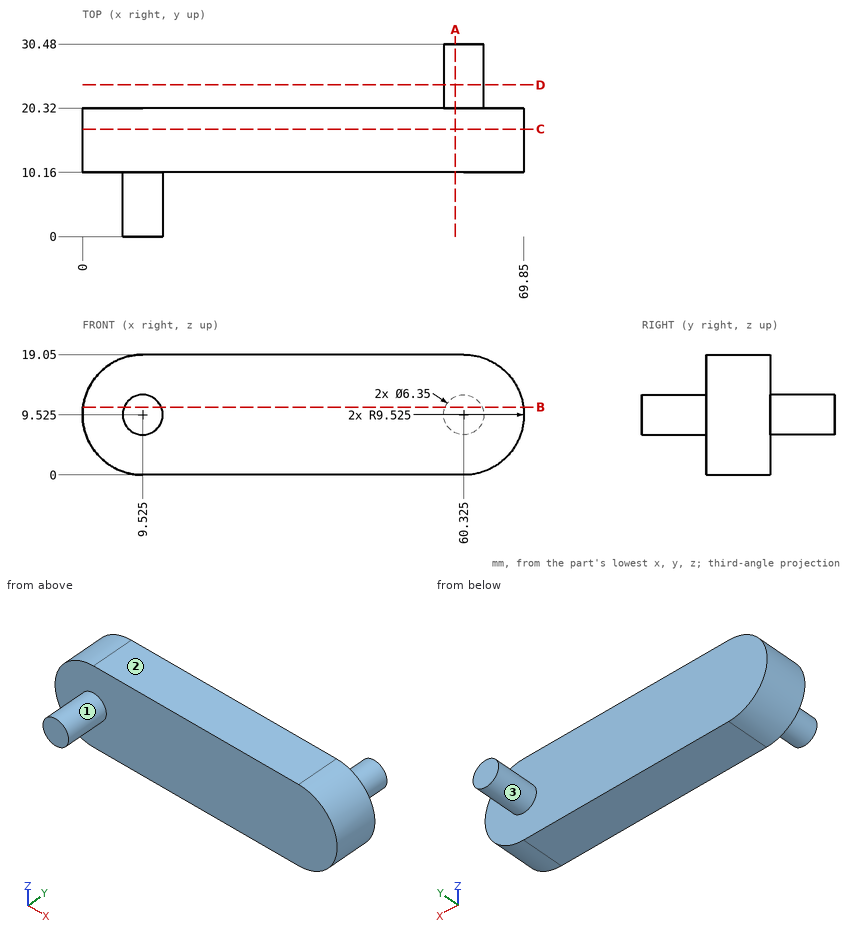
Input: dimensioned drawing with shaded views. Units: mm. Origin: part minimum x, y, z. A direction names the side the tool comes from. Coordinates: 2 decimals unless noted, no trailing zeros. Order: outer loops, then holes, each group sorted by start corner. A loop starts at its lowest first (then second) coordinate and runs counter-clockwise, first axis right, second up. Notation, with made-up numbers: (60.25, 77) -> (111.25, 77) arc R34 cw to (111.25, 112) -> close; hole circle Ø7 at (21.5, 10.25). An arc over 180 degrees is marked (long way). Use CSV: the item, a comma, the result in double quotes.
1) Line query: line 1 (Y direction, x = 21, z = 14.75); line 2 (Y direction, x = 12.5, z = 10.25); line 3 (X direction, y = 16, z = 2.5). Output: solid intervals per line, ascending.
Findings:
line 1,"y = 10.16 to 20.32"
line 2,"y = 0 to 20.32"
line 3,"x = 3.09 to 66.76"
2) Section A-A on x = 59. Output: boundary loops of the cut face in (y, z), then the cut area to 3 significant figures.
Findings:
outline,"(10.16, 0) -> (20.32, 0) -> (20.32, 6.64) -> (30.48, 6.64) -> (30.48, 12.41) -> (20.32, 12.41) -> (20.32, 19.05) -> (10.16, 19.05) -> close"
area,"252 mm^2"
3) Section D-D on y = 24. Output: boundary loops of the cut face in (x, z) (3 decimals), then the cut area to 3 significant figures.
Findings:
outline,"circle Ø6.35 at (60.325, 9.525)"
area,"31.7 mm^2"
4) Pin query (flat end, axial travel): pin 1 Ø5 at (y, z) = (7, 6) entering from +X; pin 2 Ø1 at (x, z) = (46.5, 12.5) entering from +Y. Return the tip coordinate at first contact, or that it passes through.
Findings:
pin 1,"stops at x = 12.53"
pin 2,"stops at y = 20.32"
5) Section C-C on y = 17. Output: boundary loops of the cut face in (x, z) (3 decimals), then the cut area to 3 significant figures.
Findings:
outline,"(9.525, 0) -> (60.325, 0) arc R9.525 ccw to (60.325, 19.05) -> (9.525, 19.05) arc R9.525 ccw to start"
area,"1,250 mm^2"
6) Access query for the marked faces 1, 2 and 3. Directions: +Z, -Z, +X, -X, +Y, -Y. A direction counts if a zero-diameter tool reaches every point of the face in a straight line with its end or side. Return the directions, or none.
Findings:
face 1,"-Y"
face 2,"+Z, +X, -X, +Y, -Y"
face 3,"+Y"
7) Section B-B on z = 10.75. Output: boundary loops of the cut face in (x, y).
Findings:
outline,"(0.08, 10.16) -> (6.6, 10.16) -> (6.6, 0) -> (12.45, 0) -> (12.45, 10.16) -> (69.77, 10.16) -> (69.77, 20.32) -> (63.25, 20.32) -> (63.25, 30.48) -> (57.4, 30.48) -> (57.4, 20.32) -> (0.08, 20.32) -> close"
